Here's how the part is built. I have some questions about the finished solid (model axes, mm). A direction names the side the tool comes from. Coordinates: 2 decimals unless noted, no trailing zeros. Write each loop counter-clockwise with the first axis right and the second up, starting at its lowest first coordinate (ties: lowest second). Pieces come first, ordered by that corner, then holes.
(1) Which directions (+Z, -Z, +X, -X, +Y, -Y) give clear straight access to the entire face, cutting with the end or side of a thin tool? Please do faces 1 (the cylindrical face through (-3.74, -16.84, 35.42)), 2 (the cylindrical face through (49.044, 33.627, 9.344)), 3 (the flat face through (0, 0, 50.8)).
(2) Please list where these lines run through material, in increasing order: probe 1 along Z at (x, y) = (39, -7); probe 2 along Y at (x, z) = (14, 24.5); probe 3 along Y at (x, z) = (-1.5, 25.5).
(3) Imagine slicing it at A-A, the plane x = 0. List the corners of the cut face in (y, z) for me, plus the area to 3 significant figures.
(4) For pin 1 Ø4 at (x, y) = (-10, -3) entering from -Z; pin 2 Ø1.5 at (x, z) = (5.5, 34.5) entering from -Y; pin 3 Ø5 at (x, y) = (-43.5, 6.5) entering from +Z; pin 4 Ø3 at (x, z) = (11, 21) entering from +Y, each with a flat end and sliding along its axis, tell me the tip position at first contact or that it passes through.
(5) Imagine slicing it at C-C, the plane z = 27. List the corners of the cut face in (x, y) for me.
(6) Imagine slicing it at B-B, the plane y = 0. List the corners of the cut face in (x, z) for me, plus the area to 3 significant figures.
(7) Imagine slicing it at D-D, the plane x = -38. List the corners of the cut face in (y, z) for me.
```python
from build123d import *

# Parameters (mm, degrees)
F0_W     = 124.079682
F0_H     = 55.621927
F1_DEPTH = 25.4
F2_R     = 17.251533
F3_DEPTH = 25.4
F4_R     = 5.08
F5_R     = 7.02462
F6_DEPTH = 7.62
F7_R     = 5.08


with BuildPart() as f1:
    # F0 (on Top) → F1 (new body)
    with BuildSketch(Plane.XY):
        with Locations((2.139304, 4.563851)):
            Rectangle(F0_W, F0_H)
    extrude(amount=F1_DEPTH)

    # F2 (on face) → F3 (join)
    with BuildSketch(Plane.XY.offset(25.4)):
        Circle(F2_R)
    extrude(amount=F3_DEPTH)

    # F4
    f4_edges = [f1.edges().sort_by_distance(p)[0] for p in [
        (-17.251533, 0, 50.8),
    ]]
    fillet(f4_edges, radius=F4_R)

    # F5 (on face) → F6 (join)
    with BuildSketch(Plane(origin=(0, 32.374814, 0), x_dir=(-1, 0, 0), z_dir=(0, 1, 0))):
        with Locations((-42.026419, 9.035506)):
            Circle(F5_R)
    extrude(amount=F6_DEPTH)

    # F7
    f7_edges = [f1.edges().sort_by_distance(p)[0] for p in [
        (49.051039, 39.994814, 9.035506),
    ]]
    fillet(f7_edges, radius=F7_R)


solid = f1.part
```
Recorded:
1. face 1: +Z
1. face 2: +Y
1. face 3: +Z, +X, -X, +Y, -Y
2. probe 1: z = 0 to 25.4
2. probe 2: y = -23.25 to 32.37
2. probe 3: y = -17.19 to 17.19
3. outline: (-23.25, 0) - (32.37, 0) - (32.37, 25.4) - (17.25, 25.4) - (17.25, 45.72) arc R5.08 ccw to (12.17, 50.8) - (-12.17, 50.8) arc R5.08 ccw to (-17.25, 45.72) - (-17.25, 25.4) - (-23.25, 25.4) - close
3. area: 2,280 mm2
4. pin 1: stops at z = 0
4. pin 2: stops at y = -16.58
4. pin 3: stops at z = 25.4
4. pin 4: stops at y = 32.37
5. outline: circle Ø34.5 at (0, 0)
6. outline: (-59.9, 0) - (64.18, 0) - (64.18, 25.4) - (17.25, 25.4) - (17.25, 45.72) arc R5.08 ccw to (12.17, 50.8) - (-12.17, 50.8) arc R5.08 ccw to (-17.25, 45.72) - (-17.25, 25.4) - (-59.9, 25.4) - close
6. area: 4,020 mm2
7. outline: (-23.25, 0) - (32.37, 0) - (32.37, 25.4) - (-23.25, 25.4) - close
